```python
from build123d import *

# Parameters (mm, degrees)
BOX_W           = 3
BOX_H           = 29
BOX_DEPTH       = 23
BOX001_W        = 3
BOX001_H        = 29
BOX001_DEPTH    = 23
SKETCH_R        = 1
PAD_DEPTH       = 3
SKETCH001_R     = 1.65
PAD001_DEPTH    = 1.5
PAD001_FACE17_R = 1.65
PAD002_DEPTH    = 6
PAD002_FACE15_R = 1.65
PAD003_DEPTH    = 6


with BuildPart() as box:
    # Box → Box (new body)
    with BuildSketch(Plane(origin=(1.5, -4.9, 3.1), x_dir=(1, 0, 0), z_dir=(0, 0, 1))):
        with Locations((1.5, 14.5)):
            Rectangle(BOX_W, BOX_H)
    extrude(amount=BOX_DEPTH)


with BuildPart() as box001:
    # Box001 → Box001 (new body)
    with BuildSketch(Plane(origin=(-4.5, -4.9, 3.1), x_dir=(1, 0, 0), z_dir=(0, 0, 1))):
        with Locations((1.5, 14.5)):
            Rectangle(BOX001_W, BOX001_H)
    extrude(amount=BOX001_DEPTH)


with BuildPart() as cut001:
    # Sketch → Pad (new body)
    with BuildSketch(Plane.XY):
        with BuildLine():
            Line((0, 9.082448), (10, 9.082448))
            ThreePointArc((13.264879, 2.512568), (13.6682, 6.809172), (10, 9.082448))
            Line((13.264879, 2.512568), (4.810995, -8.645152))
            ThreePointArc((0, -11.035959), (2.686151, -10.405312), (4.810995, -8.645152))
            ThreePointArc((-4.810995, -8.645152), (-2.686151, -10.405312), (0, -11.035959))
            Line((-13.264879, 2.512568), (-4.810995, -8.645152))
            ThreePointArc((-10, 9.082448), (-13.6682, 6.809172), (-13.264879, 2.512568))
            Line((0, 9.082448), (-10, 9.082448))
        make_face()
        with Locations((10, 5)):
            Circle(SKETCH_R, mode=Mode.SUBTRACT)
        with Locations((0, -5)):
            Circle(SKETCH_R, mode=Mode.SUBTRACT)
        with Locations((-10, 5)):
            Circle(SKETCH_R, mode=Mode.SUBTRACT)
    extrude(amount=PAD_DEPTH)

    # Sketch001 → Pad001 (join, symmetric)
    with BuildSketch(Plane.YZ):
        with BuildLine():
            Line((-2.970462, 2.440773), (-2.970462, 14.440773))
            ThreePointArc((9.050778, 13.866246), (3.341478, 20.458253), (-2.970462, 14.440773))
            Line((9.050778, 13.866246), (9.050778, 2.407893))
            Line((9.050778, 2.407893), (-2.970462, 2.440773))
        make_face()
        with Locations((3.053887, 14.440773)):
            Circle(SKETCH001_R, mode=Mode.SUBTRACT)
    extrude(amount=PAD001_DEPTH, both=True)

    # Pad001 Face17 → Pad002 (add)
    with BuildSketch(Plane(origin=(1.5, 3.044075, 10.994615), x_dir=(0, -1, 0), z_dir=(1, 0, 0))):
        with BuildLine():
            Line((6.014537, 7.994615), (-6.006703, 7.994615))
            Line((-6.006703, 7.994615), (-6.006703, -2.871631))
            ThreePointArc((-6.006703, -2.871631), (-0.297403, -9.463638), (6.014537, -3.446158))
            Line((6.014537, -3.446158), (6.014537, 7.994615))
        make_face()
        with Locations((-0.009812, -3.446158)):
            Circle(PAD001_FACE17_R, mode=Mode.SUBTRACT)
    extrude(amount=PAD002_DEPTH)

    # Pad002 Face15 → Pad003 (add)
    with BuildSketch(Plane(origin=(-1.5, 3.044075, 10.994615), x_dir=(0, 1, 0), z_dir=(-1, 0, 0))):
        with BuildLine():
            Line((6.006703, 7.994615), (-6.014537, 7.994615))
            Line((-6.014537, 7.994615), (-6.014537, -3.446158))
            ThreePointArc((-6.014537, -3.446158), (0.297403, -9.463638), (6.006703, -2.871631))
            Line((6.006703, -2.871631), (6.006703, 7.994615))
        make_face()
        with Locations((0.009812, -3.446158)):
            Circle(PAD002_FACE15_R, mode=Mode.SUBTRACT)
    extrude(amount=PAD003_DEPTH)

    # Cut: cut Box001
    add(box001.part, mode=Mode.SUBTRACT)

    # Cut001: cut Box
    add(box.part, mode=Mode.SUBTRACT)


solid = cut001.part
```
Check sheet for the modelled part. Datum: model origin and axes. Units: mm. A direction names the side the tool comes from. Round coordinates to 2 decimals unless told otherwise and drop trailing zeros. Write each loop counter-clockwise with the first axis right and the second up, starting at its lowest first coordinate (ties: lowest second). Pieces come first, ordered by that corner, then holes. Notation, with made-up numbers: M 37.25,35.25 L 70.25,35.25 A22 cw 70.25,73.25 Z; hole C 0.25,-23.5 d11. An arc over 180 degrees is marked long. Write item = value, one per line. Start each with the question number.
1. Section check C-C, the plane y = 3. Record the cut outline in (x, z).
2. Gauge pin test, flat ends, axial feed: pin 1 (3.5 mm diameter, centred on y = 0, z = 15.5, fed in from -X); pin 2 (1.5 mm diameter, centred on x = -3, y = 4, fed in from +Z); pin 3 (3.5 mm diameter, centred on y = 4.5, z = 7.5, fed in from +X); pin 4 (1 mm diameter, centred on x = 8.5, z = 4.5, fed in from +Y). Record the tip position at first contact, or that the pin passes through.
3. Release check for a two-part mould opening along Y. For faces 1 (the cylindrical face through (-10.737, 5.676, 1.479)), 2 (the flat face through (0, -2.97, 9)), 3 (the cylindrical face through (9.263, 5.676, 1.479)), 4 (the flat face through (0, 9.051, 8)) record: pulls with the +Y half, pulls with the -Y half, needs draft (parallel to the pull), parting line crosses it, or undercut.
4. Section check A-A, the plane z = 2.5. Record the cut outline in (x, y).
5. Section check B-B, the plane z = 7. Record the cut outline in (x, y).
6. Section check D-D, the plane y = -2.25. Record the cut outline in (x, z).
7. Scan lines: line 1 (X direction, y = 4.75, z = 4); line 2 (Z direction, x = -8.5, y = 3.75); line 3 (Y direction, x = 0.5, z = 3.75). Record each from-to range of solid material in increasing order. Write a range as [from, to].
8. Tool access check on faces 5 (the cylindrical face through (-5.979, 2.839, 12.805)), 6 (the flat face through (-1.5, 3, 12)), 7 (the flat face through (7.5, 3, 12)). Record the directions out of +Z, -Z, +X, -X, +Y, -Y that give a thin tool (end or side, any length) a straight path to the whole face; none if there is none.
Results found:
q1.outline = M -13.58,0 L 13.58,0 L 13.58,3 L 7.5,3 L 7.5,12.79 L 4.5,12.79 L 4.5,3.1 L 1.5,3.1 L 1.5,12.79 L -1.5,12.79 L -1.5,3.1 L -4.5,3.1 L -4.5,12.79 L -7.5,12.79 L -7.5,3 L -13.58,3 Z; M -7.5,16.09 L -4.5,16.09 L -4.5,20.46 L -7.5,20.46 Z; M -1.5,16.09 L 1.5,16.09 L 1.5,20.46 L -1.5,20.46 Z; M 4.5,16.09 L 7.5,16.09 L 7.5,20.46 L 4.5,20.46 Z
q2.pin_1 = -7.5
q2.pin_2 = 3.1
q2.pin_3 = 7.5
q2.pin_4 = through
q3.face_1 = undercut
q3.face_2 = pulls with the -Y half
q3.face_3 = undercut
q3.face_4 = pulls with the +Y half
q4.outline = M -13.26,2.51 L -4.81,-8.65 A6.04 ccw 0,-11.04 A6.04 ccw 4.81,-8.65 L 13.26,2.51 A4.1 ccw 10,9.08 L -10,9.08 A4.1 ccw Z; hole C -10,5 d2; hole C 0,-5 d2; hole C 10,5 d2
q5.outline = M -7.5,-2.97 L -4.5,-2.97 L -4.5,9.05 L -7.5,9.05 Z; M -1.5,-2.97 L 1.5,-2.97 L 1.5,9.05 L -1.5,9.05 Z; M 4.5,-2.97 L 7.5,-2.97 L 7.5,9.05 L 4.5,9.05 Z
q6.outline = M -9.66,0 L 9.66,0 L 9.66,3 L 7.5,3 L 7.5,17.3 L 4.5,17.3 L 4.5,3.1 L 1.5,3.1 L 1.5,17.3 L -1.5,17.3 L -1.5,3.1 L -4.5,3.1 L -4.5,17.3 L -7.5,17.3 L -7.5,3 L -9.66,3 Z
q7.line_1 = [-7.5, -4.5], [-1.5, 1.5], [4.5, 7.5]
q7.line_2 = [0, 3]
q7.line_3 = [-2.97, 9.05]
q8.face_5 = +X, -X
q8.face_6 = +Z, +Y, -Y
q8.face_7 = +Z, +X, +Y, -Y
